Part model, mm, in its own coordinate system. Give positions to 0.01 mm unless a question says otherwise; leave off trailing zeros. Write each loop counter-clockwise with the first axis right and the second up, starting at its lowest first coordinate (ties: lowest second). Pieces come first, ordered by that corner, then holes.
Solid Edge part; units mm, degrees
sketch "Sketch1" plane through (0, 0, 0) normal (0, 0, 1) x (1, 0, 0)
  line L0 (40, -15) -> (40, 15)
  line L1 (40, 15) -> (-40, 15)
  line L2 (-40, 15) -> (-40, -15)
  line L3 (-40, -15) -> (40, -15)
extrude "Protrusion1" add sketch "Sketch1" along normal blind 25
hole "Bohrung_1" at (-20, 0, 25) direction (0, 0, -1) diameter 8.5 end through all
hole "Hole1" at (20, 0, 25) direction (0, 0, -1) diameter 8.5 end through all
fillet "Verrundung_1" radius 1 4 edges at (-40, 15, 12.5) (-40, -15, 12.5) (40, -15, 12.5) (40, 15, 12.5)
1) Saw through at C-C, the plane y = 0. Write the cut outline in (x, z).
Answers follow:
outline: (-40, 0) - (-24.25, 0) - (-24.25, 25) - (-40, 25) - close; (-15.75, 0) - (15.75, 0) - (15.75, 25) - (-15.75, 25) - close; (24.25, 0) - (40, 0) - (40, 25) - (24.25, 25) - close
2) Wall check: L1, parallel to X at y = 0, z = 10.25; L2, parallel to Y at x = -20, z = 16.25; L3, parallel to X at y = 1, z = 14.25. Give the ranges that are in metal, low to high.
Answers follow:
L1: x = -40 to -24.25, -15.75 to 15.75, 24.25 to 40
L2: y = -15 to -4.25, 4.25 to 15
L3: x = -40 to -24.13, -15.87 to 15.87, 24.13 to 40
3) Saw through at B-B, the plane z = 8. Write the cut outline in (x, y).
Answers follow:
outline: (-40, -14) arc R1 ccw to (-39, -15) - (39, -15) arc R1 ccw to (40, -14) - (40, 14) arc R1 ccw to (39, 15) - (-39, 15) arc R1 ccw to (-40, 14) - close; hole circle Ø8.5 at (-20, 0); hole circle Ø8.5 at (20, 0)
4) Saw through at A-A, the plane x = 20. Write the cut outline in (y, z).
Answers follow:
outline: (-15, 0) - (-4.25, 0) - (-4.25, 25) - (-15, 25) - close; (4.25, 0) - (15, 0) - (15, 25) - (4.25, 25) - close
5) Two-plate mould, pull along X, no slides. Class faces 1 (the face through (-40, 0, 12)), 2 (the face through (-24.15, 0.92, 12.68)), 3 (the face through (-1, 0, 0)), 4 (the face through (40, 0, 12)): +X half, -X half, draft (parallel to the pull), parting line (faces both ways), or undercut.
Answers follow:
face 1: -X half
face 2: undercut
face 3: draft
face 4: +X half
